Input: part model. Units: mm. Frame: model coordinates. A direction names the side the tool comes from. Round coordinates to 2 decimals unless told otherwise and drop trailing zeros. Loops run counter-clockwise (first coordinate to the right, second up) from the corner with the lowest first, then second, coordinate; pieces in that order, holes last.
(1) Cut plane B-B, the plane x = 37.5. Output: boundary loops of the cut face in (y, z).
(2) Access query for faces 1 (the face through (44.878, -0.011, 1.521)), 2 (the face through (14.06, 16.68, 2.51)), 3 (the face through (38.71, -6.603, 1.014)), 4 (the face through (0, -7, 1)), 5 (the face through (22, -8, 2)). Directions: +Z, -Z, +X, -X, +Y, -Y. A direction counts if a zero-diameter tool reaches every point of the face in a straight line with its end or side. Return the directions, or none.
(3) Line query: line 1 (X direction, y = -7, z = 1.15); line 2 (Z direction, x = 19, y = 26.5); line 3 (Y direction, x = 37.5, z = 1.45). Output: solid intervals per line, ascending.
(4) Cut plane A-A, the plane y = -8.5. Output: boundary loops of the cut face in (x, z), and give its area (3 significant figures).
(5) Cut plane D-D, the plane y = 28. Output: boundary loops of the cut face in (x, z), and give its area (3 significant figures).
(6) Draft query along Y for faces 6 (the face through (9, 21, 2)), 7 (the face through (7.21, -6.27, 1.01)), 8 (the face through (44, -14, 1)). Return one class per face: released by +Y, released by -Y, zero draft, split by the parting line, or undercut.
(7) Cut plane C-C, the plane z = 0.8. Give the number of separate pieces and of enclosed holes in the cut face, and give its area (3 significant figures).
(8) First-contact query: pin 1 Ø6 at (x, y) = (37.5, -8.5) entering from +Z; pin 2 Ø3.5 at (x, y) = (-0.92, 10.57) entering from -Z; pin 3 Ø1.5 at (y, z) = (0, 0.5) entering from +X; pin 4 Ø0.6 at (y, z) = (-8, 1) entering from -X. Flat tips, straight axial feed; report the tip coordinate or a pass-through.
from build123d import *

# Parameters (mm, degrees)
EXTRUDE_1_DEPTH     = 3
SKETCH_2_R          = 2.25
CUT_EXTRUDE_1_DEPTH = 3
FILLET_1_R          = 5
SKETCH_3_W          = 46
SKETCH_3_H          = 15.05
CUT_EXTRUDE_2_DEPTH = 1


with BuildPart() as part:
    # ｽｹｯﾁ1 → ﾎﾞｽ - 押し出し1 (new body)
    with BuildSketch(Plane.XY):
        Polygon((17.434775789, 44.113814086), (-11.490666647, 9.641814145), (0, 0), (0, -16), (45, -16), (45, 0), (28.925442436, 34.47199994), align=None)
    extrude(amount=EXTRUDE_1_DEPTH)

    # ｽｹｯﾁ2 → ｶｯﾄ - 押し出し1 (cut)
    with BuildSketch(Plane.XY.offset(3)):
        with Locations((7.5, -8.5)):
            Circle(SKETCH_2_R)
        with Locations((-0.924426251, 10.566240396)):
            Circle(SKETCH_2_R)
        with Locations((18.35920204, 33.54757369)):
            Circle(SKETCH_2_R)
        with Locations((37.5, -8.5)):
            Circle(SKETCH_2_R)
    extrude(amount=-CUT_EXTRUDE_1_DEPTH, mode=Mode.SUBTRACT)

    # ﾌｨﾚｯﾄ1
    fillet_1_edges = [part.edges().sort_by_distance(p)[0] for p in [
        (17.434775789, 44.113814086, 1.5),
        (28.925442436, 34.47199994, 1.5),
        (45, 0, 1.5),
        (45, -16, 1.5),
        (0, -16, 1.5),
        (0, 0, 1.5),
        (-11.490666647, 9.641814145, 1.5),
    ]]
    fillet(fillet_1_edges, radius=FILLET_1_R)

    # ｽｹｯﾁ3 → ｶｯﾄ - 押し出し2 (cut)
    with BuildSketch(Plane.XY.offset(3)):
        Polygon((17.434775789, 44.113814086), (-12.133454256, 8.875769702), (-0.604485388, -0.798183824), (28.963744658, 34.43986056), align=None)
        with Locations((22, -8.475)):
            Rectangle(SKETCH_3_W, SKETCH_3_H)
    extrude(amount=-CUT_EXTRUDE_2_DEPTH, mode=Mode.SUBTRACT)


solid = part.part
Reported:
1. outline: (-16, 0) - (-10.75, 0) - (-10.75, 2) - (-16, 2) - close; (-6.25, 0) - (16.08, 0) - (16.08, 3) - (-0.95, 3) - (-0.95, 2) - (-6.25, 2) - close
2. face 1: +Z, -Z, +X, +Y
2. face 2: +Z, -X, +Y
2. face 3: +Z, -Z
2. face 4: +Z, -Z, -X, -Y
2. face 5: +Z, +X, -X, -Y
3. line 1: x = 0 to 5.82, 9.18 to 35.82, 39.18 to 45
3. line 2: z = 0 to 2
3. line 3: y = -16 to -10.75, -6.25 to 16.08
4. outline: (0, 0) - (5.25, 0) - (5.25, 2) - (0, 2) - close; (9.75, 0) - (35.25, 0) - (35.25, 2) - (9.75, 2) - close; (39.75, 0) - (45, 0) - (45, 2) - (39.75, 2) - close
4. area: 72.0 mm2
5. outline: (3.91, 0) - (31.94, 0) - (31.94, 3) - (23.56, 3) - (23.56, 2) - (3.91, 2) - close
5. area: 64.4 mm2
6. face 6: zero draft
6. face 7: undercut
6. face 8: released by -Y
7. separate pieces: 1
7. enclosed holes: 4
7. area: 2,090 mm2
8. pin 1: stops at z = 2
8. pin 2: passes through
8. pin 3: stops at x = 44.99
8. pin 4: stops at x = 0
